from build123d import *

# Parameters (mm, degrees)
SKETCH1_R           = 2.85
BOSS_EXTRUDE1_DEPTH = 3
SKETCH2_R           = 1.5
BOSS_EXTRUDE2_DEPTH = 35
CHAMFER1_SIZE       = 0.3
CUT_EXTRUDE1_DEPTH  = 2


with BuildPart() as part:
    # Sketch1 → Boss-Extrude1 (new body)
    with BuildSketch(Plane.XY):
        Circle(SKETCH1_R)
    extrude(amount=BOSS_EXTRUDE1_DEPTH)

    # Sketch2 → Boss-Extrude2 (add)
    with BuildSketch(Plane(origin=(0, 0, 0), x_dir=(-1, 0, 0), z_dir=(0, 0, -1))):
        Circle(SKETCH2_R)
    extrude(amount=BOSS_EXTRUDE2_DEPTH)

    # Chamfer1
    chamfer1_edges = [part.edges().sort_by_distance(p)[0] for p in [
        (1.5, 0, -35),
    ]]
    chamfer(chamfer1_edges, length=CHAMFER1_SIZE)

    # Sketch3 → Cut-Extrude1 (cut)
    with BuildSketch(Plane.XY.offset(3)):
        Polygon((0, 1.443375673), (-1.25, 0.721687836), (-1.25, -0.721687836), (0, -1.443375673), (1.25, -0.721687836), (1.25, 0.721687836), align=None)
    extrude(amount=-CUT_EXTRUDE1_DEPTH, mode=Mode.SUBTRACT)


solid = part.part
Verification items for the finished model (mm, model axes). A direction names the side the tool comes from. Coordinates: 2 decimals unless noted, no trailing zeros. Order: outer loops, then holes, each group sorted by start corner. A loop starts at its lowest first (then second) coordinate and runs counter-clockwise, first axis right, second up. Notation, with made-up numbers: (-25, 45) -> (31, 45) arc R23 cw to (31, 64) -> close; hole circle Ø9 at (-20.5, -34). An arc over 180 degrees is marked (long way). Put each result on its own line as item: value. Start each with the question number.
1. Access from +Z, -Z, +X, -X, +Y, -Y to the whole of each face (thin tool, end or side, straight path). Record for faces 4 (the flat face through (1.25, 0, 2)), 5 (the cylindrical face through (1.5, 0.07, -17.11)), 6 (the flat face through (-0.67, -1.23, 3)).
2. Mould release check, pull along X, two halves, no side actions. Record for faces 1 (the flat face through (0, 0, -35)), 2 (the cylindrical face through (-2.262, -1.734, 1.479)), 3 (the flat face through (0, 0, 1)): released by +X, released by -X, zero draft, split by the parting line, or undercut.
3. Cross-section at D-D, the plane y = 1.9. Record the boundary of the cut face in (x, z), then the cut area to 3 significant figures.
4. Go/stop test with flat-tipped pins: pin 1 Ø3 at (x, y) = (-0.5, -1.5) entering from -Z; pin 2 Ø1 at (x, y) = (-1, 1.5) entering from -Z; pin 3 Ø3 at (y, z) = (1, -2) entering from +X; pin 4 Ø0.7 at (y, z) = (-0.5, 2) entering from +X. Record where each tip stops, or that it passes through.
5. Material ranges on L1, parallel to Z at x = 2.2, y = 1.3; L2, parallel to Y at x = -0.05, z = -0.5; L3, parallel to X at y = -0.9, z = -23, recorded low to high. Write a range as [from, to].
6. Cross-section at B-B, the plane z = -29. Record the boundary of the cut face in (x, y).
7. Cross-section at A-A, the plane y = 0. Record the boundary of the cut face in (x, z), then the cut area to 3 significant figures.
8. Cross-section at C-C, the plane y = -2.5. Record the boundary of the cut face in (x, z), then the cut area to 3 significant figures.
Computed:
1. face 4: +Z
1. face 5: -Z
1. face 6: +Z, +X, -X, +Y, -Y
2. face 1: zero draft
2. face 2: split by the parting line
2. face 3: undercut
3. outline: (-2.12, 0) -> (2.12, 0) -> (2.12, 3) -> (-2.12, 3) -> close
3. area: 12.7 mm2
4. pin 1: z = -35
4. pin 2: z = -34.9
4. pin 3: x = 1.5
4. pin 4: x = 2.85
5. L1: [0, 3]
5. L2: [-1.5, 1.5]
5. L3: [-1.2, 1.2]
6. outline: circle Ø3 at (0, 0)
7. outline: (-2.85, 0) -> (-1.5, 0) -> (-1.5, -34.7) -> (-1.2, -35) -> (1.2, -35) -> (1.5, -34.7) -> (1.5, 0) -> (2.85, 0) -> (2.85, 3) -> (1.25, 3) -> (1.25, 1) -> (-1.25, 1) -> (-1.25, 3) -> (-2.85, 3) -> close
7. area: 117 mm2
8. outline: (-1.37, 0) -> (1.37, 0) -> (1.37, 3) -> (-1.37, 3) -> close
8. area: 8.21 mm2
